```python
from build123d import *

# Parameters (mm, degrees)
SKETCH029_R      = 35
PAD012_DEPTH     = 3
SKETCH030_R      = 15
PAD013_DEPTH     = 93
SKETCH031_R      = 18
PAD014_DEPTH     = 4
SKETCH032_R      = 7.5
POCKET010_DEPTH  = 80
SKETCH033_R      = 2
POCKET011_DEPTH  = 9
FILLET013_R      = 5
FILLET014_R      = 1
CHAMFER004_SIZE2 = 2.99
CHAMFER004_SIZE  = 5
FILLET015_R      = 2


with BuildPart() as part:
    # Sketch029 (on DatumPlane) → Pad012 (new body)
    with BuildSketch(Plane(origin=(0, 5.625, 137.8708612235), x_dir=(-1, 0, 0), z_dir=(0, -0.9781476007, 0.2079116908))):
        with Locations((-195, 18)):
            Circle(SKETCH029_R)
    extrude(amount=PAD012_DEPTH)

    # Sketch030 (on DatumPlane) → Pad013 (join)
    with BuildSketch(Plane(origin=(0, 5.625, 137.8708612235), x_dir=(-1, 0, 0), z_dir=(0, -0.9781476007, 0.2079116908))):
        with Locations((-195, 18)):
            Circle(SKETCH030_R)
    extrude(amount=PAD013_DEPTH)

    # Sketch031 (on Face6 of Pad013) → Pad014 (join)
    with BuildSketch(Plane(origin=(0, -85.3427268682, 157.2066484695), x_dir=(-1, 0, 0), z_dir=(0, -0.9781476007, 0.2079116908))):
        with Locations((-195, 18)):
            Circle(SKETCH031_R)
    extrude(amount=PAD014_DEPTH)

    # Sketch032 (on Face3 of Pad014) → Pocket010 (cut)
    with BuildSketch(Plane(origin=(0, -89.2553172712, 158.0382952328), x_dir=(-1, 0, 0), z_dir=(0, -0.9781476007, 0.2079116908))):
        with Locations((-195, 18)):
            Circle(SKETCH032_R)
    extrude(amount=-POCKET010_DEPTH, mode=Mode.SUBTRACT)

    # Sketch033 (on ReferenceDatumPlane) → Pocket011 (cut)
    with BuildSketch(Plane(origin=(0, 5.625, 137.8708612235), x_dir=(-1, 0, 0), z_dir=(0, -0.9781476007, 0.2079116908))):
        with Locations((-195, 28)):
            Circle(SKETCH033_R)
        with Locations((-185, 18)):
            Circle(SKETCH033_R)
        with Locations((-195, 8)):
            Circle(SKETCH033_R)
        with Locations((-205, 18)):
            Circle(SKETCH033_R)
    extrude(amount=POCKET011_DEPTH, mode=Mode.SUBTRACT)

    # Fillet013
    fillet013_edges = [part.edges().sort_by_distance(p)[0] for p in [
        (210, -1.051853, 120.887939),
        (202.5, -92.997728, 140.431638),
    ]]
    fillet(fillet013_edges, radius=FILLET013_R)

    # Fillet014
    fillet014_edges = [part.edges().sort_by_distance(p)[0] for p in [
        (230, -1.051853, 120.887939),
    ]]
    fillet(fillet014_edges, radius=FILLET014_R)

    # Chamfer004
    chamfer004_edges = [part.edges().sort_by_distance(p)[0] for p in [
        (210, -89.085137, 139.599992),
    ]]
    chamfer004_side = part.faces().sort_by_distance((210, -47.513864, 130.763745))[0]
    chamfer(chamfer004_edges, length=CHAMFER004_SIZE, length2=CHAMFER004_SIZE2, reference=chamfer004_side)

    # Fillet015
    fillet015_edges = [part.edges().sort_by_distance(p)[0] for p in [
        (213, -92.997728, 140.431638),
    ]]
    fillet(fillet015_edges, radius=FILLET015_R)


solid = part.part
```
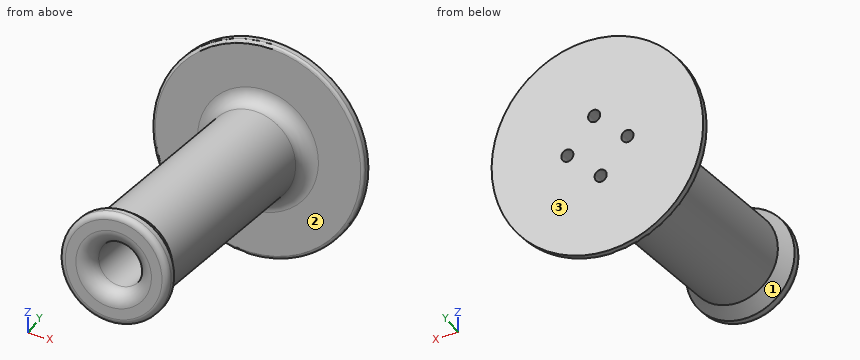
Check sheet for the modelled part. Datum: model origin and axes. Units: mm. Face numbers are marked on the shaded views. Coordinates: 2 decimals unless noted, no trailing zeros. Write each question's results on one line, items separated by ' | '. Start each with the question number.
1. Mould release check, pull along Z, two halves, no side actions. Record for the marked faces 1, 2 and 3: +Z half, -Z half, draft (parallel to the pull), parting line (faces both ways), or undercut.
2. Go/stop test with flat-tipped pins: P1, Ø2, axis at y = -45, z = 134, coming from the -X side; P2, Ø4, axis at x = 219, z = 98, coming from the +Y side; P3, Ø6, axis at x = 198.5, y = -11, coming from the +Z side. Record where each tip stops, or that it passes through.
3. Material ranges on probe 1 along Z at (x, y) = (199, -53.5); probe 2 along Y at (x, z) = (181.5, 148); probe 3 along Z at (x, y) = (196.5, -44.5), recorded low to high.
Checks:
1) face 1: parting line | face 2: undercut | face 3: -Z half
2) P1: stops at x = 180.24 | P2: stops at y = -2.42 | P3: stops at z = 138.75
3) probe 1: z = 117.26 to 125.55, 138.52 to 146.82 | probe 2: y = -91.39 to -84.45, 4.71 to 7.78 | probe 3: z = 114.86 to 122.61, 137.64 to 145.38
